```python
from build123d import *

# Parameters (mm, degrees)
BOSS_EXTRUDE1_DEPTH = 2.5


with BuildPart() as part:
    # frame_outline → Boss-Extrude1 (new, symmetric)
    with BuildSketch(Plane.XY):
        Polygon((0, 0), (0, 0.25), (3, 0.25), (2.625519601, 3.130114195), (3.311145122, 3.558555133), (6.555598399, 1.109884861), (6.792166473, 1.257714025), (6.792166473, 4.533228245), (7.259759156, 4.825422514), (9.729524263, 3.356316312), (10.341620659, 3.738809591), (10.341620659, 5.671508671), (10.591620659, 5.671508671), (10.591620659, 3.600234825), (9.732731436, 3.063523029), (7.262966329, 4.532629231), (7.042166473, 4.394653478), (7.042166473, 1.119139258), (6.542252093, 0.806747465), (3.297798816, 3.255417737), (2.894129781, 3.003168755), (3.284610073, 0), (3, 0), align=None)
    extrude(amount=BOSS_EXTRUDE1_DEPTH, both=True)


solid = part.part
```
Verification items for the finished model (mm, model axes). A direction names the side the tool comes from. Round coordinates to 2 decimals unless told otherwise and drop trailing zeros. Write each loop counter-clockwise with the first axis right and the second up, starting at its lowest first coordinate (ties: lowest second). Pieces come first, ordered by that corner, then holes.
1. Draft check along Y on faces 1 (the flat face through (7.042, 3, 0)), 2 (the flat face through (8.48, 4.1, 0.04)), 3 (the flat face through (3.087, 1.523, 0.035)). Enter one of: +Y half, -Y half, draft (parallel to the pull), parting line (faces both ways), or undercut.
2. Scan lines: L1, parallel to X at y = 1.6, z = -1.9; L2, parallel to X at y = 2, z = -1.95; L3, parallel to Y at x = 2.25, z = -2.15. Record each from-to range of solid material in increasing order.
3. Section check B-B on z = -2. Enter the section's corners in (x, y).
4. Section check C-C on x = 9.25. Enter the section's corners in (y, z), plus the area to 3 significant figures.
5. Access from +Z, -Z, +X, -X, +Y, -Y to the whole of each face (thin tool, end or side, straight path). Record for faces 4 (the flat face through (4.943, 2.014, 0.035)), 5 (the flat face through (6.792, 3, 0)), 6 (the flat face through (2.815, 1.67, 0.035)), 7 (the flat face through (2, 0, 0)).
6. Section check A-A on y = 1.8. Enter the section's corners in (x, z).
7. Section check D-D on y = 4.95. Enter the section's corners in (x, z).
8. Gauge pin test, flat ends, axial feed: P1, Ø2, axis at y = 1, z = 1.5, coming from the -X side; P2, Ø2, axis at x = 3, z = -0.5, coming from the +Y side; P3, Ø2.5, axis at y = 3, z = -0.5, coming from the -X side; P4, Ø1, axis at x = 4.5, z = 1.5, coming from the -Y side. Record the tip position at first contact, or that the pin passes through.
Answer:
1. face 1: draft
1. face 2: +Y half
1. face 3: undercut
2. L1: x = 2.82 to 3.08, 5.49 to 5.91, 6.79 to 7.04
2. L2: x = 2.77 to 3.02, 4.96 to 5.38, 6.79 to 7.04
2. L3: y = 0 to 0.25
3. outline: (0, 0) - (3.28, 0) - (2.89, 3) - (3.3, 3.26) - (6.54, 0.81) - (7.04, 1.12) - (7.04, 4.39) - (7.26, 4.53) - (9.73, 3.06) - (10.59, 3.6) - (10.59, 5.67) - (10.34, 5.67) - (10.34, 3.74) - (9.73, 3.36) - (7.26, 4.83) - (6.79, 4.53) - (6.79, 1.26) - (6.56, 1.11) - (3.31, 3.56) - (2.63, 3.13) - (3, 0.25) - (0, 0.25) - close
4. outline: (3.35, -2.5) - (3.64, -2.5) - (3.64, 2.5) - (3.35, 2.5) - close
4. area: 1.45 mm2
5. face 4: +Z, -Z, -Y
5. face 5: +Z, -Z, +Y
5. face 6: +Z, -Z, -X
5. face 7: +Z, -Z, +X, -X, -Y
6. outline: (2.8, -2.5) - (3.05, -2.5) - (3.05, 2.5) - (2.8, 2.5) - close; (5.23, -2.5) - (5.64, -2.5) - (5.64, 2.5) - (5.23, 2.5) - close; (6.79, -2.5) - (7.04, -2.5) - (7.04, 2.5) - (6.79, 2.5) - close
7. outline: (10.34, -2.5) - (10.59, -2.5) - (10.59, 2.5) - (10.34, 2.5) - close
8. P1: stops at x = 0
8. P2: stops at y = 3.56
8. P3: stops at x = 2.63
8. P4: stops at y = 1.97
